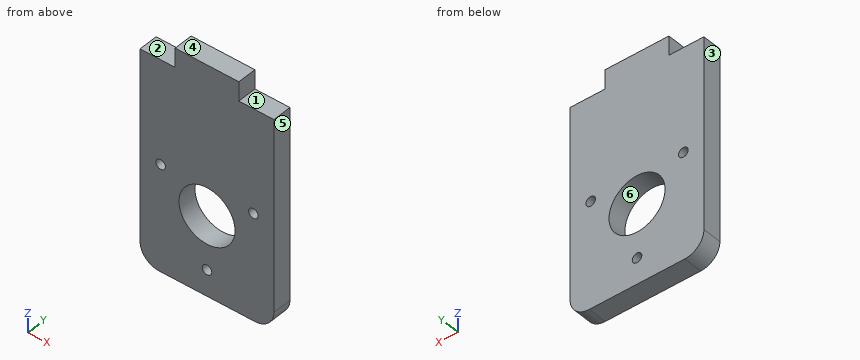
```python
from build123d import *

# Parameters (mm, degrees)
ESQUISSE1_R        = 4.4
ESQUISSE1_R_2      = 0.75
BOSS_EXTRU_1_DEPTH = 3


with BuildPart() as part:
    # Esquisse1 → Boss.-Extru.1 (new body)
    with BuildSketch(Plane(origin=(0, 0, 0), x_dir=(1, 0, 0), z_dir=(0, 1, 0))):
        with BuildLine():
            Line((-10.5, 3), (-5, 3))
            Line((-5, 3), (-5, 0))
            Line((-5, 0), (5, 0))
            Line((5, 0), (5, 3))
            Line((5, 3), (10.5, 3))
            Line((10.5, 3), (10.5, 33))
            ThreePointArc((10.5, 33), (9.621320344, 35.121320344), (7.5, 36))
            Line((7.5, 36), (-7.5, 36))
            ThreePointArc((-7.5, 36), (-9.621320344, 35.121320344), (-10.5, 33))
            Line((-10.5, 33), (-10.5, 3))
        make_face()
        with Locations(Location((0, 23.5, 0), (0, 0, 270))):
            Circle(ESQUISSE1_R, mode=Mode.SUBTRACT)
        with Locations(Location((0, 31.9, 0), (0, 0, 270))):
            Circle(ESQUISSE1_R_2, mode=Mode.SUBTRACT)
        with Locations(Location((7.274613392, 19.3, 0), (0, 0, 270))):
            Circle(ESQUISSE1_R_2, mode=Mode.SUBTRACT)
        with Locations(Location((-7.274613392, 19.3, 0), (0, 0, 270))):
            Circle(ESQUISSE1_R_2, mode=Mode.SUBTRACT)
    extrude(amount=BOSS_EXTRU_1_DEPTH)


solid = part.part
```
Design review of the part built by this model. Coordinates are the model's own, in mm. Face numbers are marked on the shaded views. A direction names the side the tool comes from. Give positions to 0.01 mm unless a question says otherwise; leave off trailing zeros. Order: outer loops, then holes, each group sorted by start corner. A loop starts at its lowest first (then second) coordinate and runs counter-clockwise, first axis right, second up. Notation, with made-up numbers: (76.25, -10.5) -> (132.25, -10.5) arc R9 ccw to (132.25, 5.5) -> close; hole circle Ø4 at (8.5, 19). An arc over 180 degrees is marked (long way). Write item = value, one per line. Start each with the question number.
(1) For pin 1 (0.9 mm diameter, centred on x = 7.27, z = -19.3, fed in from -Y), flat-tipped, find the tip position at first contact; note if it passes through.
(2) We need section C-C on y = 2.5. Write out the cut boundary in (x, z).
(3) We need section A-A on x = 0. Write out the cut boundary in (y, z).
(4) Mouldability with a two-part tool opening along X and no side actions: class the marked faces 4, 5 and 6 as +X half, -X half, draft (parallel to the pull), parting line (faces both ways), or undercut.
(5) We need section B-B on z = -31.9. Write out the cut boundary in (x, y), plus the area to 3 significant figures.
(6) For the marked faces 1, 2 and 3, list the 3-axis set-ups (+Z, -Z, +X, -X, +Y, -Y) from which the entire face can be reached by the end or side of a thin tool; tool diameter is ignored.
(7) We need section D-D on x = -2.75. Write out the cut boundary in (y, z), plus the area to 3 significant figures.
(8) To check wall thickness, follow line 1 along X through (y, z) = (1, -31.9); line 2 along X through (y, z) = (1.4, -23.5); line 3 along Z through (x, y) = (6, 1). State the ranges of each line that lie inside material, in increasing order.
Numbers:
q1.pin_1 = through
q2.outline = (-10.5, -33) arc R3 ccw to (-7.5, -36) -> (7.5, -36) arc R3 ccw to (10.5, -33) -> (10.5, -3) -> (5, -3) -> (5, 0) -> (-5, 0) -> (-5, -3) -> (-10.5, -3) -> close; hole circle Ø1.5 at (-7.27, -19.3); hole circle Ø8.8 at (0, -23.5); hole circle Ø1.5 at (0, -31.9); hole circle Ø1.5 at (7.27, -19.3)
q3.outline = (0, -36) -> (3, -36) -> (3, -32.65) -> (0, -32.65) -> close; (0, -31.15) -> (3, -31.15) -> (3, -27.9) -> (0, -27.9) -> close; (0, -19.1) -> (3, -19.1) -> (3, 0) -> (0, 0) -> close
q4.face_4 = draft
q4.face_5 = +X half
q4.face_6 = undercut
q5.outline = (-10.5, 0) -> (-0.75, 0) -> (-0.75, 3) -> (-10.5, 3) -> close; (0.75, 0) -> (10.5, 0) -> (10.5, 3) -> (0.75, 3) -> close
q5.area = 58.5 mm^2
q6.face_1 = +Z, +X, +Y, -Y
q6.face_2 = +Z, -X, +Y, -Y
q6.face_3 = +Z, -Z, -X, +Y, -Y
q7.outline = (0, -36) -> (3, -36) -> (3, -26.93) -> (0, -26.93) -> close; (0, -20.07) -> (3, -20.07) -> (3, 0) -> (0, 0) -> close
q7.area = 87.4 mm^2
q8.line_1 = -10.5 to -0.75, 0.75 to 10.5
q8.line_2 = -10.5 to -4.4, 4.4 to 10.5
q8.line_3 = -36 to -3
